Geometry: final body of the model. Coordinates: model frame, mm. Face numbers are marked on the shaded views. A direction names the side the tool comes from. Give positions to 0.01 mm unless a question says otherwise; leave off trailing zeros. Write each loop counter-clockwise with the first axis right and the second up, starting at its lowest first coordinate (ties: lowest second). Pieces come first, ordered by that corner, then holes. Notation, with made-up numbers: (61.5, 70) - (98.5, 70) arc R20 cw to (98.5, 108) - close; hole circle Ø1 at (38.25, 86.5). An arc over 180 degrees is marked (long way). Use CSV: the item, a comma, the result in double quotes. Start each with the question number.
(1) Reachability of the marked faces 1 and 2 from +Z, -Z, +X, -X, +Y, -Y: full face, straight path, thin tool, end or side. Return the list, or none.
(2) Section B-B on y = 10. Output: boundary loops of the cut face in (x, z), and give its area (3 significant figures).
(3) Section D-D on z = -14.25. Output: boundary loops of the cut face in (x, y).
(4) Section C-C on z = -10. Output: boundary loops of the cut face in (x, y), and give its area (3 significant figures).
(5) Line query: probe 1 along X at (y, z) = (-22.75, -10); probe 2 along X at (y, z) = (-22, -14.32); probe 3 along X at (y, z) = (10, 1). Output: solid intervals per line, ascending. Write a range as [from, to].
(6) First-contact query: pin 1 Ø5 at (x, z) = (5.5, -8.5) entering from +Y; pin 2 Ø2 at (y, z) = (1.5, 2) entering from -X; pin 3 Ø19 at (x, y) = (-13, 10) entering from +Z; pin 4 Ø1.5 at (y, z) = (-2.5, -2) entering from -X. Flat tips, straight axial feed; report the tip coordinate or a pass-through.
(7) Section A-A on x = 4.71. Output: boundary loops of the cut face in (y, z).
from build123d import *

# Parameters (mm, degrees)
EXTRUDE_1_DEPTH     = 3
SKETCH_2_W          = 27
SKETCH_2_H          = 3
EXTRUDE_2_DEPTH     = 20
FILLET_1_SIZE       = 3
FILLET_2_SIZE       = 3
SKETCH_3_R          = 2.5
SKETCH_3_R_2        = 0.75
CUT_EXTRUDE_1_DEPTH = 20
SKETCH_4_R          = 1
CUT_EXTRUDE_2_DEPTH = 10


with BuildPart() as part:
    # 草图1 → 凸台-拉伸1 (new body)
    with BuildSketch(Plane.XY):
        with BuildLine():
            Line((-10, 23), (-21.14797242, 23))
            ThreePointArc((-21.14797242, 23), (-22.380603493, 22.735072328), (-23.395529179, 21.987080425))
            Line((-23.395529179, 21.987080425), (-26.168091228, 18.851077224))
            ThreePointArc((-26.168091228, 18.851077224), (-26.72612445, 17.926383199), (-26.920534469, 16.863996799))
            Line((-26.920534469, 16.863996799), (-26.920534469, 6.136003201))
            ThreePointArc((-26.920534469, 6.136003201), (-26.72612445, 5.073616801), (-26.168091228, 4.148922776))
            Line((-26.168091228, 4.148922776), (-22.5, 0))
            Line((-22.5, 0), (-14.378679656, -8.121320344))
            ThreePointArc((-14.378679656, -8.121320344), (-13.728361402, -9.09459039), (-13.5, -10.242640687))
            Line((-13.5, -10.242640687), (-13.5, -24))
            Line((-13.5, -24), (13.5, -24))
            Line((13.5, -24), (13.5, -10.242640687))
            ThreePointArc((13.5, -10.242640687), (13.728361402, -9.09459039), (14.378679656, -8.121320344))
            Line((14.378679656, -8.121320344), (22.5, 0))
            Line((22.5, 0), (26.168091228, 4.148922776))
            ThreePointArc((26.168091228, 4.148922776), (26.72612445, 5.073616801), (26.920534469, 6.136003201))
            Line((26.920534469, 6.136003201), (26.920534469, 16.863996799))
            ThreePointArc((26.920534469, 16.863996799), (26.72612445, 17.926383199), (26.168091228, 18.851077224))
            Line((26.168091228, 18.851077224), (23.395529179, 21.987080425))
            ThreePointArc((23.395529179, 21.987080425), (22.380603493, 22.735072328), (21.14797242, 23))
            Line((21.14797242, 23), (10, 23))
            Line((10, 23), (-10, 23))
        make_face()
        with BuildLine():
            Line((-10, 20), (10, 20))
            Line((10, 20), (10, 17.685213074))
            ThreePointArc((10, 17.685213074), (21.245514188, 9.727978361), (9.5, 2.529223601))
            Line((9.5, 2.529223601), (9.5, 0))
            Line((9.5, 0), (-9.5, 0))
            Line((-9.5, 0), (-9.5, 2.529223601))
            ThreePointArc((-9.5, 2.529223601), (-21.245514188, 9.727978361), (-10, 17.685213074))
            Line((-10, 17.685213074), (-10, 20))
        make_face(mode=Mode.SUBTRACT)
    extrude(amount=EXTRUDE_1_DEPTH)

    # 草图2 → 凸台-拉伸2 (add)
    with BuildSketch(Plane(origin=(0, 0, 0), x_dir=(-1, 0, 0), z_dir=(0, 0, -1))):
        with Locations((0, -22.5)):
            Rectangle(SKETCH_2_W, SKETCH_2_H)
    extrude(amount=EXTRUDE_2_DEPTH)

    # 圆角1
    # a fillet whose section is not a circle: 3 mm, written as the material it takes off along each edge
    with BuildSketch(Plane(origin=(13.5, -31.5, -20), x_dir=(-1, 0, 0), z_dir=(0, 1, 0))) as fillet_1_piece_1:
        with BuildLine():
            add(Edge.make_bspline([(FILLET_1_SIZE, 0), (FILLET_1_SIZE * 0.831801948466, 0), (FILLET_1_SIZE * 0.663603896932, 0), (FILLET_1_SIZE * 0.292893218813, FILLET_1_SIZE * 0.0716919198361), (FILLET_1_SIZE * 0.0716919198361, FILLET_1_SIZE * 0.292893218813), (0, FILLET_1_SIZE * 0.663603896932), (0, FILLET_1_SIZE * 0.831801948466), (0, FILLET_1_SIZE)], knots=[0, 0, 0, 0, 0, 0, 0.5, 0.5, 1, 1, 1, 1, 1, 1], degree=5))
            Line((0, FILLET_1_SIZE), (0, 0))
            Line((0, 0), (FILLET_1_SIZE, 0))
        make_face()
    extrude(amount=18, mode=Mode.SUBTRACT)

    # 圆角2
    # a fillet whose section is not a circle: 3 mm, written as the material it takes off along each edge
    with BuildSketch(Plane(origin=(-13.5, -13.5, -20), x_dir=(0, 0, 1), z_dir=(0, -1, 0))) as fillet_2_piece_1:
        with BuildLine():
            add(Edge.make_bspline([(FILLET_2_SIZE, 0), (FILLET_2_SIZE * 0.831801948466, 0), (FILLET_2_SIZE * 0.663603896932, 0), (FILLET_2_SIZE * 0.292893218813, -FILLET_2_SIZE * 0.0716919198361), (FILLET_2_SIZE * 0.0716919198361, -FILLET_2_SIZE * 0.292893218813), (0, -FILLET_2_SIZE * 0.663603896932), (0, -FILLET_2_SIZE * 0.831801948466), (0, -FILLET_2_SIZE)], knots=[0, 0, 0, 0, 0, 0, 0.5, 0.5, 1, 1, 1, 1, 1, 1], degree=5))
            Line((0, -FILLET_2_SIZE), (0, 0))
            Line((0, 0), (FILLET_2_SIZE, 0))
        make_face()
    extrude(amount=18, mode=Mode.SUBTRACT)

    # 草图3 → 切除-拉伸1 (cut)
    with BuildSketch(Plane(origin=(0, -21, 0), x_dir=(1, 0, 0), z_dir=(0, 1, 0))):
        with Locations(Location((0, 10, 0), (0, 0, 270))):
            Circle(SKETCH_3_R)
        with Locations(Location((-4.71, 10, 0), (0, 0, 270))):
            Circle(SKETCH_3_R_2)
        with Locations(Location((0, 14.32, 0), (0, 0, 270))):
            Circle(SKETCH_3_R_2)
        with Locations(Location((0, 5.68, 0), (0, 0, 270))):
            Circle(SKETCH_3_R_2)
        with Locations(Location((4.71, 10, 0), (0, 0, 270))):
            Circle(SKETCH_3_R_2)
    extrude(amount=-CUT_EXTRUDE_1_DEPTH, mode=Mode.SUBTRACT)

    # 草图4 → 切除-拉伸2 (cut)
    with BuildSketch(Plane.XY.offset(3)):
        with Locations((-21.255, 18.855)):
            Circle(SKETCH_4_R)
        with Locations((-21.255, 1.145)):
            Circle(SKETCH_4_R)
        with Locations((21.255, 18.855)):
            Circle(SKETCH_4_R)
        with Locations((21.255, 1.145)):
            Circle(SKETCH_4_R)
    extrude(amount=-CUT_EXTRUDE_2_DEPTH, mode=Mode.SUBTRACT)


solid = part.part
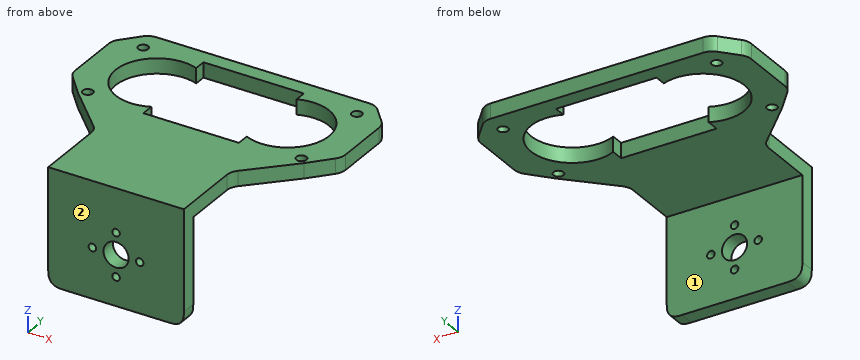
Check values:
1,face 1,"-Z, +X, -X, +Y"
1,face 2,"+Z, -Z, +X, -X, -Y"
2,outline,"(-26.92, 0) - (-21.25, 0) - (-21.25, 3) - (-26.92, 3) - close; (21.25, 0) - (26.92, 0) - (26.92, 3) - (21.25, 3) - close"
2,area,"34.0 mm²"
3,outline,"(-13.5, -24) - (-0.75, -24) - (-0.75, -21) - (-13.5, -21) - close; (0.75, -24) - (13.5, -24) - (13.5, -21) - (0.75, -21) - close"
4,outline,"(-13.5, -24) - (-5.46, -24) - (-5.46, -21) - (-13.5, -21) - close; (-3.96, -24) - (-2.5, -24) - (-2.5, -21) - (-3.96, -21) - close; (2.5, -24) - (3.96, -24) - (3.96, -21) - (2.5, -21) - close; (5.46, -24) - (13.5, -24) - (13.5, -21) - (5.46, -21) - close"
4,area,"57.0 mm²"
5,probe 1,"x = [-13.5, -5.46], [-3.96, -2.5], [2.5, 3.96], [5.46, 13.5]"
5,probe 2,"x = [-13.5, -0.75], [0.75, 13.5]"
5,probe 3,"x = [-26.92, -21.25], [21.25, 26.92]"
6,pin 1,"stops at y = -21"
6,pin 2,"stops at x = -24.71"
6,pin 3,"stops at z = 3"
6,pin 4,"passes through"
7,outline,"(-24, -20) - (-21, -20) - (-21, -10.75) - (-24, -10.75) - close; (-24, -9.25) - (-21, -9.25) - (-21, 0) - (0, 0) - (0, 3) - (-24, 3) - close; (20, 0) - (23, 0) - (23, 3) - (20, 3) - close"
